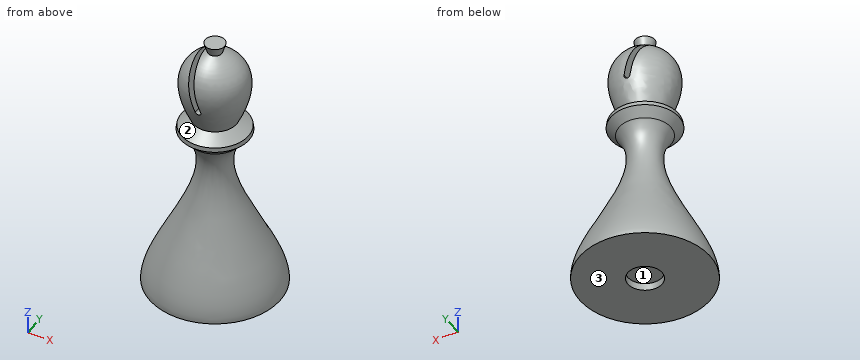
Autodesk Fusion 360 part; units mm, degrees
sketch "Sketch1" plane through (0, 0, 0) normal (0, 1, 0) x (1, 0, 0)
  line L0 (0, 0) -> (0, -80)
  line L1 (0, 0) -> (-20, 0)
  line L2 (-6.0501, -55.2545) -> (-10.2637, -52.2049)
  line L3 (-10.4525, -50.8951) -> (-5.4129, -45.8555)
  line L4 (-10.2637, -52.2049) -> (-10.4525, -50.8951)
  line L5 (0, -70.5202) -> (-2.9993, -80)
  line L6 (-2.9993, -80) -> (0, -80)
  spline S0 degree 5 poles (-20, 0) (-20, -0.6734) (-19.8627, -2.1332) (-19.2448, -4.6616) (-17.6673, -8.6584) (-14.8349, -14.4044) (-11.653, -20.5245) (-8.6578, -26.6258) (-6.3321, -32.3545) (-5.0054, -37.4666) (-4.7896, -41.8717) (-5.5103, -44.8202) (-6.5359, -46.7178) (-7.4317, -47.8457) (-7.9327, -48.3753) knots 0 0 0 0 0 0 0.1 0.2 0.3 0.4 0.5 0.6 0.7 0.8 0.9 1 1 1 1 1 1
  spline S1 degree 5 poles (-6.6133, -54.8469) (-6.9485, -55.5323) (-7.579, -56.8841) (-8.4052, -58.855) (-9.2635, -61.3672) (-9.9029, -64.3011) (-10.0667, -67.0089) (-9.7113, -69.4697) (-8.8041, -71.6681) (-7.3543, -73.6084) (-5.3976, -75.3076) (-3.4574, -76.4886) (-1.8044, -77.2803) (-0.6159, -77.767) (0, -78) knots 0 0 0 0 0 0 0.1 0.2 0.3 0.4 0.5 0.6 0.7 0.8 0.9 1 1 1 1 1 1
  line L7 (-20, 3) -> (-20, -3)
  line L8 (-5.25, 0) -> (-5.25, -2.25)
  line L9 (-5.25, -2.25) -> (0, -2.25)
  point P0 (-7, -31)
  point P1 (-9.3943, -69.9909)
  dimension "d2" = 20
  dimension "d5" = 80
  dimension "d7" = 45
  dimension "d8" = 2.25
  dimension "d9" = 5.25
revolve "Revolve1" add sketch "Sketch1" angle 360 about axis through (0, 0, 0) along (0, 0, 1) contours L0 L1 L2 L3 L4 L5 S0 S1 L8 L9 | L0 L5 S1 | L0 L5 L6 S1
sketch "Sketch2" plane through (0, 0, 0) normal (0, 1, 0) x (1, 0, 0)
  line L0 (-5.5, -78) -> (-0.7405, -62.5113)
  line L1 (-0.7405, -62.5113) -> (1.027, -63.0544)
  line L2 (1.027, -63.0544) -> (-3.8706, -78.9928)
  arc A0 (1.027, -63.0544) -> (-0.7405, -62.5113) centre (0.1432, -62.7828) ccw
  line L3 (-5.5, -78) -> (-3.8706, -78.9928)
extrude "Extrude1" cut sketch "Sketch2" along normal through all and the other way through all
equation "d2 = d1 * 1 / 4"
Build history of the part. All positions in model axes, mm. Face numbers are marked on the shaded views. Coordinates: 2 decimals unless noted, no trailing zeros. Write each loop counter-clockwise with the first axis right and the second up, starting at its lowest first coordinate (ties: lowest second). Pieces come first, ordered by that corner, then holes.
(1) Cut at A-A on z = 50. List the corners of the cut face in (x, y), and give its area (3 significant figures).
(2) Mould opens along Y. For the marked faces 1, 2 and 3 say: pulls with the +Y half, pulls with the -Y half, needs draft (parallel to the pull), parting line crosses it, or undercut.
(3) Pin check, flat tips, straight feed: pin 1 Ø8 at (y, z) = (-5.5, 34) entering from -X; pin 2 Ø1.5 at (x, y) = (-5, 6.5) entering from +Z; pin 3 Ø1 at (x, y) = (-12.5, 9.5) entering from +Z. Stop position of each tip, or through.
(4) Drill centre lines: line 1 (Y direction, x = 0, z = 0.55); line 2 (X direction, y = 0, z = 1.7); line 3 (Y direction, x = 0, z = 1). Where is each one in solid material? Low to high.
Working result:
1. outline: circle Ø19.11 at (0, 0)
1. area: 287 mm2
2. face 1: undercut
2. face 2: parting line crosses it
2. face 3: needs draft
3. pin 1: stops at x = -6.4
3. pin 2: stops at z = 73.3
3. pin 3: stops at z = 13.59
4. line 1: y = -19.98 to -5.25, 5.25 to 19.98
4. line 2: x = -19.85 to -5.25, 5.25 to 19.85
4. line 3: y = -19.94 to -5.25, 5.25 to 19.94
